Autodesk Inventor part; units mm, degrees
ref_plane "YZ Plane" through (0, 0, 0) normal (1, 0, 0) x (0, 1, 0)
ref_plane "XZ Plane" through (0, 0, 0) normal (0, 1, 0) x (-1, 0, 0)
ref_plane "XY Plane" through (0, 0, 0) normal (0, 0, 1) x (1, 0, 0)
sketch "Sketch1" plane through (0, 0, 0) normal (0, 0, 1) x (1, 0, 0)
  line L0 (-431.8, -266.7) -> (431.8, -266.7)
  line L1 (431.8, -266.7) -> (431.8, 266.7)
  line L2 (431.8, 266.7) -> (-431.8, 266.7)
  line L3 (-431.8, 266.7) -> (-431.8, -266.7)
  line L4 (-431.8, -266.7) -> (431.8, 266.7) construction
  line L5 (431.8, -266.7) -> (-431.8, 266.7) construction
  point P0 (0, 0)
  dimension "d0" = 863.6
  dimension "d1" = 533.4
extrude "Extrusion1" add sketch "Sketch1" along normal blind 152.4
sketch "Sketch2" plane through (431.8, -266.7, 0) normal (1, 0, 0) x (0, 0, -1)
  line L0 (0, 0) -> (0, 533.4)
  line L1 (0, 0) -> (-152.4, 0)
  arc A0 (0, 387.7039) -> (0, 501.2961) centre (-50.8, 444.5) ccw
  line L2 (0, 266.7) -> (-335.0591, 266.7) construction
  line L3 (0, 501.2961) -> (0, 387.7039)
  arc A1 (0, 32.1039) -> (0, 145.6961) centre (-50.8, 88.9) ccw
  line L4 (0, 32.1039) -> (0, 145.6961)
extrude "Extrusion2" add sketch "Sketch2" against normal blind 76.2
extrude "Extrusion3" cut sketch "Sketch2" against normal blind 50.8
sketch "Sketch3" plane through (-431.8, -266.7, 0) normal (-1, 0, 0) x (0, 0, 1)
  line L0 (0, 501.2961) -> (0, 387.7039)
  arc A0 (0, 501.2961) -> (0, 387.7039) centre (50.8, 444.5) ccw
  line L1 (0, 145.6961) -> (0, 32.1039)
  arc A1 (0, 145.6961) -> (0, 32.1039) centre (50.8, 88.9) ccw
  point P0 (0, 266.7)
extrude "Extrusion4" add sketch "Sketch3" against normal blind 76.2
extrude "Extrusion5" cut sketch "Sketch3" against normal blind 50.8
sketch "Sketch4" plane through (0, 0, 152.4) normal (0, 0, 1) x (1, 0, 0)
  line L0 (-419.1, -254) -> (419.1, -254)
  line L1 (419.1, -254) -> (419.1, 254)
  line L2 (419.1, 254) -> (-419.1, 254)
  line L3 (-419.1, 254) -> (-419.1, -254)
  line L4 (-419.1, -254) -> (419.1, 254) construction
  line L5 (419.1, -254) -> (-419.1, 254) construction
  point P0 (0, 0)
  dimension "d14" = 838.2
  dimension "d15" = 508
extrude "Extrusion6" cut sketch "Sketch4" against normal blind 139.7
sketch "Sketch5" plane through (0, 0, 12.7) normal (0, 0, 1) x (1, 0, 0)
  line L0 (203.2, -50.8) -> (177.8, -50.8)
  line L1 (177.8, -50.8) -> (177.8, 50.8)
  line L2 (177.8, 50.8) -> (203.2, 50.8)
  line L3 (203.2, 50.8) -> (203.2, -50.8)
  line L4 (203.2, -50.8) -> (177.8, 50.8) construction
  line L5 (177.8, -50.8) -> (203.2, 50.8) construction
  line L6 (-203.2, -50.8) -> (-177.8, -50.8)
  line L7 (-177.8, -50.8) -> (-177.8, 50.8)
  line L8 (-177.8, 50.8) -> (-203.2, 50.8)
  line L9 (-203.2, 50.8) -> (-203.2, -50.8)
  point P0 (0, 0)
  dimension "d19" = 25.4
  dimension "d20" = 101.6
extrude "Extrusion7" add sketch "Sketch5" along normal blind 609.6
sketch "Sketch6" plane through (203.2, -50.8, 12.7) normal (1, 0, 0) x (0, 0, -1)
  line L0 (-609.6, 0) -> (-609.6, 101.6)
  line L1 (0, 0) -> (-609.6, 0)
  line L2 (-609.6, 50.8) -> (-304.8, 50.8)
  point P0 (12.7, 50.8)
  dimension "d23" = 304.8
hole "Hole1" at (203.2, 0, 317.5) direction (-1, 0, 0) diameter 12.7 end through all
sketch "Sketch7" plane through (0, 0, 152.4) normal (0, 0, 1) x (1, 0, 0)
  line L0 (-431.8, -266.7) -> (431.8, -266.7)
  line L1 (0, -266.7) -> (228.6, -266.7)
  line L2 (228.6, -266.7) -> (228.6, -186.436)
  line L3 (228.6, -186.436) -> (-228.6, -186.436)
  line L4 (-228.6, -186.436) -> (-228.6, -266.7)
  line L5 (0, -266.7) -> (-228.6, -266.7)
  point P0 (0, 0)
  dimension "d31" = 228.6
  dimension "d32" = 80.264
  dimension "d33" = 457.2
extrude "Extrusion8" cut sketch "Sketch7" against normal through all
properties part number "Base"
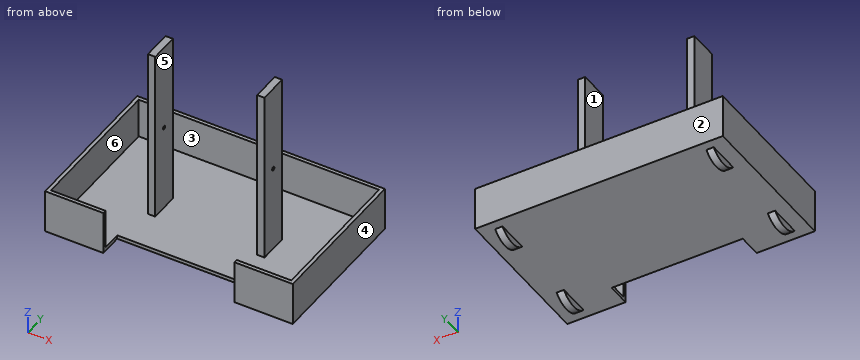
The model under review builds one solid part; all positions refer to its coordinate system, in mm. Face numbers are marked on the shaded views. A direction names the side the tool comes from. Coordinates: 2 decimals unless noted, no trailing zeros. Order: outer loops, then holes, each group sorted by start corner. A loop starts at its lowest first (then second) coordinate and runs counter-clockwise, first axis right, second up. Notation, with made-up numbers: (75, 82.25) -> (133, 82.25) arc R24 ccw to (133, 93.25) -> close; hole circle Ø5 at (44, 72). An arc over 180 degrees is marked (long way). Answer in a Markdown table with one row per item.
(1) Consider section C-C (y = 169). Write out the cut boundary in (x, z), plus the area to 3 significant figures.
Answers:
| item | result |
|---|---|
| outline | (-431.8, 0) -> (-381, 0) -> (-381, -24.89) -> (-355.6, -24.89) -> (-355.6, 0) -> (355.6, 0) -> (355.6, -24.89) -> (381, -24.89) -> (381, 0) -> (431.8, 0) -> (431.8, 152.4) -> (419.1, 152.4) -> (419.1, 12.7) -> (-419.1, 12.7) -> (-419.1, 152.4) -> (-431.8, 152.4) -> close |
| area | 15,800 mm² |
(2) Insertion check: pin 1 (1 mm diameter, centred on x = 199, y = -148.5, fed in from +Z); pin 2 (12.5 mm diameter, centred on x = 192, z = 184, fed in from +Y); pin 3 (20.5 mm diameter, centred on y = -200.5, z = -14, fed in from +X). Each pin has a flat end and moves straight along its axis. Give the tip position at first contact, or say it passes through.
Answers:
| item | result |
|---|---|
| pin 1 | z = 12.7 |
| pin 2 | y = 50.8 |
| pin 3 | x = 381 |
(3) Consider section B-B (x = -188). Write out the cut boundary in (y, z), plus the area to 3 significant figures.
Answers:
| item | result |
|---|---|
| outline | (-186.44, 0) -> (266.7, 0) -> (266.7, 152.4) -> (254, 152.4) -> (254, 12.7) -> (50.8, 12.7) -> (50.8, 622.3) -> (-50.8, 622.3) -> (-50.8, 12.7) -> (-186.44, 12.7) -> close; hole circle Ø12.7 at (0, 317.5) |
| area | 69,300 mm² |
(4) Wall thickness on line 1 along X through (y, z) = (7.5, 96.5); line 2 along X through (y, z) = (197, 18.5); line 3 along Z through (x, y) = (196, 0): over which ranges is each line inside the solid? List them lowest first.
Answers:
| item | result |
|---|---|
| line 1 | -431.8 to -419.1, -203.2 to -177.8, 177.8 to 203.2, 419.1 to 431.8 |
| line 2 | -431.8 to -419.1, 419.1 to 431.8 |
| line 3 | 0 to 311.15, 323.85 to 622.3 |
(5) Consider section D-D (x = -275.5). Write out the cut boundary in (y, z), plus the area to 3 significant figures.
Answers:
| item | result |
|---|---|
| outline | (-266.7, 0) -> (266.7, 0) -> (266.7, 152.4) -> (254, 152.4) -> (254, 12.7) -> (-254, 12.7) -> (-254, 152.4) -> (-266.7, 152.4) -> close |
| area | 10,300 mm² |
(6) Consider section A-A (z = 531). Write out the cut boundary in (x, y), plus the area to 3 significant figures.
Answers:
| item | result |
|---|---|
| outline | (-203.2, -50.8) -> (-177.8, -50.8) -> (-177.8, 50.8) -> (-203.2, 50.8) -> close; (177.8, -50.8) -> (203.2, -50.8) -> (203.2, 50.8) -> (177.8, 50.8) -> close |
| area | 5,160 mm² |
(7) Machinability: for the marked faces 4, 5 and 6, which of the approach directions +Z, -Z, +X, -X, +Y, -Y give a long, thin tool a straight path to every point of the face, cutting with its end or side? Answer none if there is none.
Answers:
| item | result |
|---|---|
| face 4 | +Z, -Z, +X, +Y, -Y |
| face 5 | +Z, -Y |
| face 6 | +Z |
(8) The part is to be moulded in two halves that separate along Y. For the marked faces 1, 2 and 3, say which applies: +Y half, -Y half, draft (parallel to the pull), parting line (faces both ways), or undercut.
Answers:
| item | result |
|---|---|
| face 1 | draft |
| face 2 | +Y half |
| face 3 | undercut |
